The listing builds one solid part. Answer for the finished solid, in the listing's coordinates (mm). Face numbers are marked on the shaded views. A direction names the side the tool comes from. Round coordinates to 2 decimals unless told otherwise and drop trailing zeros. Write each loop counter-clockwise with the first axis right and the second up, starting at its lowest first coordinate (ties: lowest second). Pieces come first, ordered by that corner, then holes. Notation, with made-up numbers: (65.25, 71.25) - (97.25, 71.25) arc R21 ccw to (97.25, 84.25) - close; hole circle Ø5 at (17, 62.25). An arc over 180 degrees is marked (long way). Return JSON: item names as keys, results as strings. Group by question number.
(1) Each of these flat-tipped pins is pushed along its axis until it touches: pin 1 (1 mm diameter, centred on x = 9.5, z = 34, fed in from +Y); pin 2 (1 mm diameter, centred on x = 9.5, y = 55.5, fed in from +Z); pin 3 (3.5 mm diameter, centred on y = 9.6, z = 28.25, fed in from +X); pin 4 (10 mm diameter, centred on y = 21, z = 17.5, fed in from -X). Where does it stop, or does it pass through?
(2) Which of the six approach directions +Z, -Z, +X, -X, +Y, -Y give full straight-line access (tool end or side, diameter ignored) to the marked faces 3 and 4?
(3) Section A-A, the plane z = 25.7 is taken. Write down the section's boundary in (x, y).
(4) Find the intervals of material crossed by line 1 along Y through (x, z) = (13.15, 5.3); line 2 along Y through (x, z) = (12, 13.5); line 3 along Z through (x, y) = (13.15, 49.6), in increasing order. Write a range as [from, to].
(5) Determine the mould class of the marked faces 1 and 2 for opening direction Z: +Z half, -Z half, draft (parallel to the pull), parting line (faces both ways), or undercut.
(6) Section B-B, the plane y = 13.5 is taken. Write down the section's boundary in (x, z).
(7) Section C-C, the plane z = 10 is taken. Write down the section's boundary in (x, y) (3 decimals).
(8) Section D-D, the plane x = 9.75 is taken. Write down the section's boundary in (y, z), then the cut area to 3 significant figures.
```python
from build123d import *

# Parameters (mm, degrees)
BASE_DEPTH               = 80
SCREW_HOLES_BASE_REACH   = 4
SKETCH3_R                = 1.75
SKETCH6_W                = 31
SKETCH6_H                = 38.5
SKETCH6_W_2              = 27
SKETCH6_H_2              = 34.5
S2MINI_DEPTH             = 1
SKETCH8_R                = 1.75
SCREW_HOLES_S2MINI_DEPTH = 10
SKETCH10_W               = 31
SKETCH10_H               = 23.5
SKETCH10_W_2             = 27
SKETCH10_H_2             = 19.5
MD_DEPTH                 = 1
SKETCH12_R               = 1.15
SCREW_HOLES_MD_DEPTH     = 10
SKETCH14_W               = 25.6
SKETCH14_H               = 47.6
SKETCH14_W_2             = 21.6
SKETCH14_H_2             = 43.6
BC_DEPTH                 = 1
SKETCH16_R               = 1.5
SCREW_HOLES_BC_DEPTH     = 10
SKETCH17_W               = 20
SKETCH17_H               = 27
SKETCH17_W_2             = 18
SKETCH17_H_2             = 25
LA_DEPTH                 = 1
CUT_EXTRUDE6_REACH       = 3
SKETCH18_R               = 1.75


with BuildPart() as part:
    # Sketch1 → Base (new body)
    with BuildSketch(Plane.XY):
        Polygon((0, 0), (0, 2), (12.55, 2), (12.55, 80), (13.55, 80), (13.55, 0), align=None)
    extrude(amount=BASE_DEPTH)

    # Sketch3 → Screw_Holes_Base (cut, up to next)
    with BuildSketch(Plane(origin=(0, 2, 0), x_dir=(1, 0, 0), z_dir=(0, 1, 0)), mode=Mode.PRIVATE) as screw_holes_base_sk1:
        with Locations((6.275, -10)):
            Circle(SKETCH3_R)
    screw_holes_base_tool1 = extrude(screw_holes_base_sk1.sketch, amount=-SCREW_HOLES_BASE_REACH, mode=Mode.PRIVATE) & part.part
    add(screw_holes_base_tool1.solids().sort_by_distance((6.275, 2, 10))[0], mode=Mode.SUBTRACT)
    # Sketch3 → Screw_Holes_Base (cut, up to next)
    with BuildSketch(Plane(origin=(0, 2, 0), x_dir=(1, 0, 0), z_dir=(0, 1, 0)), mode=Mode.PRIVATE) as screw_holes_base_sk2:
        with Locations((6.275, -70)):
            Circle(SKETCH3_R)
    screw_holes_base_tool2 = extrude(screw_holes_base_sk2.sketch, amount=-SCREW_HOLES_BASE_REACH, mode=Mode.PRIVATE) & part.part
    add(screw_holes_base_tool2.solids().sort_by_distance((6.275, 2, 70))[0], mode=Mode.SUBTRACT)

    # Sketch6 → S2Mini (add)
    with BuildSketch(Plane(origin=(12.55, -16.871702151, -147.313128111), x_dir=(0, 0, 1), z_dir=(-1, 0, 0))):
        with Locations((162.813128111, 77.621702151)):
            Rectangle(SKETCH6_W, SKETCH6_H)
        with Locations((162.813128111, 77.621702151)):
            Rectangle(SKETCH6_W_2, SKETCH6_H_2, mode=Mode.SUBTRACT)
    extrude(amount=S2MINI_DEPTH)

    # Sketch8 → Screw_Holes_S2Mini (cut)
    with BuildSketch(Plane(origin=(12.55, 0, 13.55), x_dir=(0, 0, -1), z_dir=(1, 0, 0))):
        with Locations((-12.15, 75.4)):
            Circle(SKETCH8_R)
        with Locations((8.25, 75.4)):
            Circle(SKETCH8_R)
        with Locations((-12.15, 49.6)):
            Circle(SKETCH8_R)
        with Locations((8.25, 49.6)):
            Circle(SKETCH8_R)
    extrude(amount=SCREW_HOLES_S2MINI_DEPTH, mode=Mode.SUBTRACT)

    # Sketch10 → MD (add)
    with BuildSketch(Plane(origin=(12.55, 37.151538962, -62.266989531), x_dir=(0, 0, 1), z_dir=(-1, 0, 0))):
        with Locations((124.766989531, -20.401538962)):
            Rectangle(SKETCH10_W, SKETCH10_H)
        with Locations((124.766989531, -20.401538962)):
            Rectangle(SKETCH10_W_2, SKETCH10_H_2, mode=Mode.SUBTRACT)
    md = extrude(amount=MD_DEPTH)

    # Sketch12 → Screw_Holes_MD (cut)
    with BuildSketch(Plane(origin=(12.55, 0, 13.55), x_dir=(0, 0, -1), z_dir=(1, 0, 0))):
        with Locations((-59.7, 9.6)):
            Circle(SKETCH12_R)
        with Locations((-38.2, 9.6)):
            Circle(SKETCH12_R)
    screw_holes_md = extrude(amount=SCREW_HOLES_MD_DEPTH, mode=Mode.SUBTRACT)

    # Mirror1: MD, Screw_Holes_MD across plane
    add(md.mirror(Plane.XY.offset(40)))
    add(screw_holes_md.mirror(Plane.XY.offset(40)), mode=Mode.SUBTRACT)

    # Sketch14 → BC (add)
    with BuildSketch(Plane(origin=(12.55, 28.832330024, -107.15387648), x_dir=(0, 0, 1), z_dir=(-1, 0, 0))):
        with Locations((174.35387648, 27.367669976)):
            Rectangle(SKETCH14_W, SKETCH14_H)
        with Locations((174.35387648, 27.367669976)):
            Rectangle(SKETCH14_W_2, SKETCH14_H_2, mode=Mode.SUBTRACT)
    extrude(amount=BC_DEPTH)

    # Sketch16 → Screw_Holes_BC (cut)
    with BuildSketch(Plane(origin=(12.55, 0, 13.55), x_dir=(0, 0, -1), z_dir=(1, 0, 0))):
        with Locations((-45.45, 40.5)):
            Circle(SKETCH16_R)
        with Locations((-61.85, 71.9)):
            Circle(SKETCH16_R)
    extrude(amount=SCREW_HOLES_BC_DEPTH, mode=Mode.SUBTRACT)

    # Sketch17 → LA (add)
    with BuildSketch(Plane.ZY.offset(-12.55)):
        with Locations((42.7, 63.5)):
            Rectangle(SKETCH17_W, SKETCH17_H)
        with Locations((42.7, 63.5)):
            Rectangle(SKETCH17_W_2, SKETCH17_H_2, mode=Mode.SUBTRACT)
    extrude(amount=LA_DEPTH)

    # Sketch18 → Cut-Extrude6 (cut, up to next)
    with BuildSketch(Plane.ZY.offset(-12.55), mode=Mode.PRIVATE) as cut_extrude6_sk1:
        with Locations((36.2, 73.5)):
            Circle(SKETCH18_R)
    cut_extrude6_tool1 = extrude(cut_extrude6_sk1.sketch, amount=-CUT_EXTRUDE6_REACH, mode=Mode.PRIVATE) & part.part
    add(cut_extrude6_tool1.solids().sort_by_distance((12.55, 73.5, 36.2))[0], mode=Mode.SUBTRACT)
    # Sketch18 → Cut-Extrude6 (cut, up to next)
    with BuildSketch(Plane.ZY.offset(-12.55), mode=Mode.PRIVATE) as cut_extrude6_sk2:
        with Locations((49.2, 73.5)):
            Circle(SKETCH18_R)
    cut_extrude6_tool2 = extrude(cut_extrude6_sk2.sketch, amount=-CUT_EXTRUDE6_REACH, mode=Mode.PRIVATE) & part.part
    add(cut_extrude6_tool2.solids().sort_by_distance((12.55, 73.5, 49.2))[0], mode=Mode.SUBTRACT)


solid = part.part
```
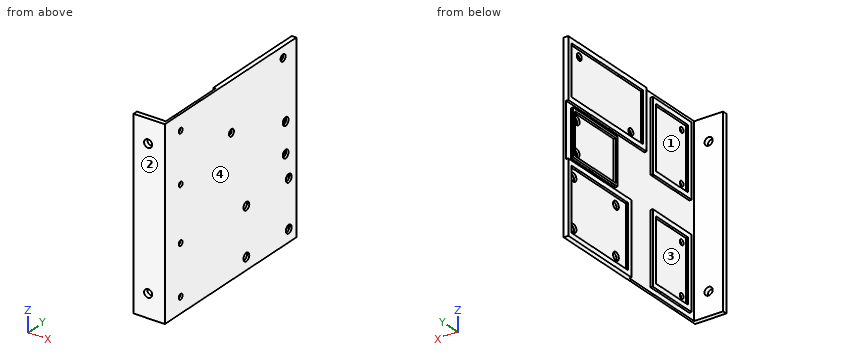
Working result:
{
 "1": {"pin 1": "stops at y = 2", "pin 2": "passes through", "pin 3": "stops at x = 13.55", "pin 4": "stops at x = 12.55"},
 "2": {"face 3": "-X", "face 4": "+Z, -Z, +X, +Y, -Y"},
 "3": {"outline": "(0, 0) - (13.55, 0) - (13.55, 47.85) - (12.55, 47.85) - (12.55, 43.5) - (11.55, 43.5) - (11.55, 41.5) - (12.55, 41.5) - (12.55, 28.5) - (11.55, 28.5) - (11.55, 26.5) - (12.55, 26.5) - (12.55, 7) - (11.55, 7) - (11.55, 5) - (12.55, 5) - (12.55, 2) - (0, 2) - close; (11.55, 78) - (12.55, 78) - (12.55, 77.15) - (13.55, 77.15) - (13.55, 80) - (11.55, 80) - close; (12.55, 51.35) - (13.55, 51.35) - (13.55, 73.65) - (12.55, 73.65) - close"},
 "4": {"line 1": "y = [0, 47.85], [51.35, 73.65], [77.15, 80]", "line 2": "y = [0, 2], [5, 7], [26.5, 28.5], [41.5, 43.5], [78, 80]", "line 3": "z = [0, 3.55], [7.05, 23.95], [27.45, 80]"},
 "5": {"face 1": "undercut", "face 2": "draft"},
 "6": {"outline": "(11.55, 2) - (12.55, 2) - (12.55, 0) - (13.55, 0) - (13.55, 80) - (12.55, 80) - (12.55, 78) - (11.55, 78) - (11.55, 76) - (12.55, 76) - (12.55, 49) - (11.55, 49) - (11.55, 47) - (12.55, 47) - (12.55, 33) - (11.55, 33) - (11.55, 31) - (12.55, 31) - (12.55, 4) - (11.55, 4) - close"},
 "7": {"outline": "(0, 0) - (4.525, 0) - (4.525, 2) - (0, 2) - close; (8.025, 0) - (13.55, 0) - (13.55, 80) - (11.55, 80) - (11.55, 78) - (12.55, 78) - (12.55, 43.5) - (11.55, 43.5) - (11.55, 41.5) - (12.55, 41.5) - (12.55, 28.5) - (11.55, 28.5) - (11.55, 26.5) - (12.55, 26.5) - (12.55, 7) - (11.55, 7) - (11.55, 5) - (12.55, 5) - (12.55, 2) - (8.025, 2) - close"},
 "8": {"outline": "(0, 0) - (2, 0) - (2, 80) - (0, 80) - close", "area": "160 mm^2"}
}
